from build123d import *

# Parameters (mm, degrees)
BOX021_W     = 19
BOX021_H     = 2
BOX021_DEPTH = 7
BOX020_W     = 19
BOX020_H     = 2
BOX020_DEPTH = 7
BOX018_W     = 1.5
BOX018_H     = 1.5
BOX018_DEPTH = 11.5
BOX016_W     = 1.5
BOX016_H     = 1.5
BOX016_DEPTH = 11.5
BOX017_W     = 1.5
BOX017_H     = 1.5
BOX017_DEPTH = 11.5
BOX019_W     = 1.5
BOX019_H     = 1.5
BOX019_DEPTH = 11.5
BOX015_W     = 5
BOX015_H     = 5
BOX015_DEPTH = 10
BOX013_W     = 1.5
BOX013_H     = 1.5
BOX013_DEPTH = 11.5
BOX011_W     = 1.5
BOX011_H     = 1.5
BOX011_DEPTH = 11.5
BOX012_W     = 1.5
BOX012_H     = 1.5
BOX012_DEPTH = 11.5
BOX014_W     = 1.5
BOX014_H     = 1.5
BOX014_DEPTH = 11.5
BOX010_W     = 5
BOX010_H     = 5
BOX010_DEPTH = 10
BOX023_W     = 19
BOX023_H     = 2
BOX023_DEPTH = 7
BOX003_W     = 1.5
BOX003_H     = 1.5
BOX003_DEPTH = 11.5
BOX001_W     = 1.5
BOX001_H     = 1.5
BOX001_DEPTH = 11.5
BOX002_W     = 1.5
BOX002_H     = 1.5
BOX002_DEPTH = 11.5
BOX004_W     = 1.5
BOX004_H     = 1.5
BOX004_DEPTH = 11.5
BOX_W        = 5
BOX_H        = 5
BOX_DEPTH    = 10
BOX008_W     = 1.5
BOX008_H     = 1.5
BOX008_DEPTH = 11.5
BOX006_W     = 1.5
BOX006_H     = 1.5
BOX006_DEPTH = 11.5
BOX007_W     = 1.5
BOX007_H     = 1.5
BOX007_DEPTH = 11.5
BOX009_W     = 1.5
BOX009_H     = 1.5
BOX009_DEPTH = 11.5
BOX005_W     = 5
BOX005_H     = 5
BOX005_DEPTH = 10
BOX024_W     = 2
BOX024_H     = 3
BOX024_DEPTH = 4
BOX022_W     = 19
BOX022_H     = 2
BOX022_DEPTH = 7


with BuildPart() as cubo021:
    # Box021 → Box021 (new body)
    with BuildSketch(Plane(origin=(0, 5.5, 0), x_dir=(1, 0, 0), z_dir=(0, 0, 1))):
        with Locations((9.5, 1)):
            Rectangle(BOX021_W, BOX021_H)
    extrude(amount=BOX021_DEPTH)


with BuildPart() as cubo020:
    # Box020 → Box020 (new body)
    with BuildSketch(Plane(origin=(18, -10.5, 0), x_dir=(0, 1, 0), z_dir=(0, 0, 1))):
        with Locations((9.5, 1)):
            Rectangle(BOX020_W, BOX020_H)
    extrude(amount=BOX020_DEPTH)


with BuildPart() as cubo018:
    # Box018 → Box018 (new body)
    with BuildSketch(Plane(origin=(3.5, 3.5, 0), x_dir=(1, 0, 0), z_dir=(0, 0, 1))):
        with Locations((0.75, 0.75)):
            Rectangle(BOX018_W, BOX018_H)
    extrude(amount=BOX018_DEPTH)


with BuildPart() as cubo016:
    # Box016 → Box016 (new body)
    with BuildSketch(Plane(origin=(0, 3.5, 0), x_dir=(1, 0, 0), z_dir=(0, 0, 1))):
        with Locations((0.75, 0.75)):
            Rectangle(BOX016_W, BOX016_H)
    extrude(amount=BOX016_DEPTH)


with BuildPart() as cubo017:
    # Box017 → Box017 (new body)
    with BuildSketch(Plane(origin=(3.5, 0, 0), x_dir=(1, 0, 0), z_dir=(0, 0, 1))):
        with Locations((0.75, 0.75)):
            Rectangle(BOX017_W, BOX017_H)
    extrude(amount=BOX017_DEPTH)


with BuildPart() as cubo019:
    # Box019 → Box019 (new body)
    with BuildSketch(Plane.XY):
        with Locations((0.75, 0.75)):
            Rectangle(BOX019_W, BOX019_H)
    extrude(amount=BOX019_DEPTH)


with BuildPart() as fusion015:
    # Box015 → Box015 (new body)
    with BuildSketch(Plane.XY):
        with Locations((2.5, 2.5)):
            Rectangle(BOX015_W, BOX015_H)
    extrude(amount=BOX015_DEPTH)

    # Fusion012: union Cubo019
    add(cubo019.part)

    # Fusion013: union Cubo017
    add(cubo017.part)

    # Fusion014: union Cubo016
    add(cubo016.part)

    # Fusion015: union Cubo018
    add(cubo018.part)


with BuildPart() as fusion015_1:
    # Fusion015 placement: moved
    add(fusion015.part.moved(Location((14, 4, 0))))


with BuildPart() as cubo013:
    # Box013 → Box013 (new body)
    with BuildSketch(Plane(origin=(3.5, 3.5, 0), x_dir=(1, 0, 0), z_dir=(0, 0, 1))):
        with Locations((0.75, 0.75)):
            Rectangle(BOX013_W, BOX013_H)
    extrude(amount=BOX013_DEPTH)


with BuildPart() as cubo011:
    # Box011 → Box011 (new body)
    with BuildSketch(Plane(origin=(0, 3.5, 0), x_dir=(1, 0, 0), z_dir=(0, 0, 1))):
        with Locations((0.75, 0.75)):
            Rectangle(BOX011_W, BOX011_H)
    extrude(amount=BOX011_DEPTH)


with BuildPart() as cubo012:
    # Box012 → Box012 (new body)
    with BuildSketch(Plane(origin=(3.5, 0, 0), x_dir=(1, 0, 0), z_dir=(0, 0, 1))):
        with Locations((0.75, 0.75)):
            Rectangle(BOX012_W, BOX012_H)
    extrude(amount=BOX012_DEPTH)


with BuildPart() as cubo014:
    # Box014 → Box014 (new body)
    with BuildSketch(Plane.XY):
        with Locations((0.75, 0.75)):
            Rectangle(BOX014_W, BOX014_H)
    extrude(amount=BOX014_DEPTH)


with BuildPart() as fusion011:
    # Box010 → Box010 (new body)
    with BuildSketch(Plane.XY):
        with Locations((2.5, 2.5)):
            Rectangle(BOX010_W, BOX010_H)
    extrude(amount=BOX010_DEPTH)

    # Fusion008: union Cubo014
    add(cubo014.part)

    # Fusion009: union Cubo012
    add(cubo012.part)

    # Fusion010: union Cubo011
    add(cubo011.part)

    # Fusion011: union Cubo013
    add(cubo013.part)


with BuildPart() as fusion011_1:
    # Fusion011 placement: moved
    add(fusion011.part.moved(Location((14, -11, 0))))


with BuildPart() as cubo023:
    # Box023 → Box023 (new body)
    with BuildSketch(Plane(origin=(4, -10.5, 0), x_dir=(0, 1, 0), z_dir=(0, 0, 1))):
        with Locations((9.5, 1)):
            Rectangle(BOX023_W, BOX023_H)
    extrude(amount=BOX023_DEPTH)


with BuildPart() as cubo003:
    # Box003 → Box003 (new body)
    with BuildSketch(Plane(origin=(3.5, 3.5, 0), x_dir=(1, 0, 0), z_dir=(0, 0, 1))):
        with Locations((0.75, 0.75)):
            Rectangle(BOX003_W, BOX003_H)
    extrude(amount=BOX003_DEPTH)


with BuildPart() as cubo001:
    # Box001 → Box001 (new body)
    with BuildSketch(Plane(origin=(0, 3.5, 0), x_dir=(1, 0, 0), z_dir=(0, 0, 1))):
        with Locations((0.75, 0.75)):
            Rectangle(BOX001_W, BOX001_H)
    extrude(amount=BOX001_DEPTH)


with BuildPart() as cubo002:
    # Box002 → Box002 (new body)
    with BuildSketch(Plane(origin=(3.5, 0, 0), x_dir=(1, 0, 0), z_dir=(0, 0, 1))):
        with Locations((0.75, 0.75)):
            Rectangle(BOX002_W, BOX002_H)
    extrude(amount=BOX002_DEPTH)


with BuildPart() as cubo004:
    # Box004 → Box004 (new body)
    with BuildSketch(Plane.XY):
        with Locations((0.75, 0.75)):
            Rectangle(BOX004_W, BOX004_H)
    extrude(amount=BOX004_DEPTH)


with BuildPart() as fusion003:
    # Box → Box (new body)
    with BuildSketch(Plane.XY):
        with Locations((2.5, 2.5)):
            Rectangle(BOX_W, BOX_H)
    extrude(amount=BOX_DEPTH)

    # Fusion: union Cubo004
    add(cubo004.part)

    # Fusion001: union Cubo002
    add(cubo002.part)

    # Fusion002: union Cubo001
    add(cubo001.part)

    # Fusion003: union Cubo003
    add(cubo003.part)


with BuildPart() as fusion003_1:
    # Fusion003 placement: moved
    add(fusion003.part.moved(Location((0, 4, 0))))


with BuildPart() as cubo008:
    # Box008 → Box008 (new body)
    with BuildSketch(Plane(origin=(3.5, 3.5, 0), x_dir=(1, 0, 0), z_dir=(0, 0, 1))):
        with Locations((0.75, 0.75)):
            Rectangle(BOX008_W, BOX008_H)
    extrude(amount=BOX008_DEPTH)


with BuildPart() as cubo006:
    # Box006 → Box006 (new body)
    with BuildSketch(Plane(origin=(0, 3.5, 0), x_dir=(1, 0, 0), z_dir=(0, 0, 1))):
        with Locations((0.75, 0.75)):
            Rectangle(BOX006_W, BOX006_H)
    extrude(amount=BOX006_DEPTH)


with BuildPart() as cubo007:
    # Box007 → Box007 (new body)
    with BuildSketch(Plane(origin=(3.5, 0, 0), x_dir=(1, 0, 0), z_dir=(0, 0, 1))):
        with Locations((0.75, 0.75)):
            Rectangle(BOX007_W, BOX007_H)
    extrude(amount=BOX007_DEPTH)


with BuildPart() as cubo009:
    # Box009 → Box009 (new body)
    with BuildSketch(Plane.XY):
        with Locations((0.75, 0.75)):
            Rectangle(BOX009_W, BOX009_H)
    extrude(amount=BOX009_DEPTH)


with BuildPart() as fusion007:
    # Box005 → Box005 (new body)
    with BuildSketch(Plane.XY):
        with Locations((2.5, 2.5)):
            Rectangle(BOX005_W, BOX005_H)
    extrude(amount=BOX005_DEPTH)

    # Fusion004: union Cubo009
    add(cubo009.part)

    # Fusion005: union Cubo007
    add(cubo007.part)

    # Fusion006: union Cubo006
    add(cubo006.part)

    # Fusion007: union Cubo008
    add(cubo008.part)


with BuildPart() as fusion007_1:
    # Fusion007 placement: moved
    add(fusion007.part.moved(Location((0, -11, 0))))


with BuildPart() as cubo024:
    # Box024 → Box024 (new body)
    with BuildSketch(Plane(origin=(8.5, -10, 0), x_dir=(1, 0, 0), z_dir=(0, 0, 1))):
        with Locations((1, 1.5)):
            Rectangle(BOX024_W, BOX024_H)
    extrude(amount=BOX024_DEPTH)


with BuildPart() as fusion016:
    # Box022 → Box022 (new body)
    with BuildSketch(Plane(origin=(0, -9.5, 0), x_dir=(1, 0, 0), z_dir=(0, 0, 1))):
        with Locations((9.5, 1)):
            Rectangle(BOX022_W, BOX022_H)
    extrude(amount=BOX022_DEPTH)

    # Cut: cut Cubo024
    add(cubo024.part, mode=Mode.SUBTRACT)

    # Fusion016: union Cubo021, Cubo020, Fusion015, Fusion011, Cubo023, Fusion003, Fusion007
    add(cubo021.part)
    add(cubo020.part)
    add(fusion015_1.part)
    add(fusion011_1.part)
    add(cubo023.part)
    add(fusion003_1.part)
    add(fusion007_1.part)


solid = fusion016.part
Here's how the part is built. I have some questions about the finished solid (model axes, mm). A direction names the side the tool comes from. Round coordinates to 2 decimals unless told otherwise and drop trailing zeros. Write each loop counter-clockwise with the first axis right and the second up, starting at its lowest first coordinate (ties: lowest second). Pieces come first, ordered by that corner, then holes.
1. Suppose I cut it at A-A (y = 2.5). List the corners of the cut face in (x, z) for me, and give its area (3 significant figures).
2. I need wall thicknesses on L1, parallel to X at y = -5.75, z = 4.25; L2, parallel to Y at x = 15, z = 2.5; L3, parallel to Y at x = 8.25, z = 3. Which ranges of each line are inside material? Lowest first, please.
3. If we mould it in two halves opening along Y, with no side actions, what happens to faces 1 (the flat face through (9, -9, 7)), 2 (the flat face through (15, 7.5, 11)), 3 (the flat face through (2, -11, 6))? For each: released by +Y, released by -Y, zero draft, split by the parting line, or undercut.
4. Will these pins go through, and if not, where does the flat tip stop? pin 1 Ø1.5 at (y, z) = (5.5, 3.5) entering from -X; pin 2 Ø1.5 at (x, y) = (16, 6.5) entering from +Z; pin 3 Ø2 at (x, z) = (8.5, 3.5) entering from -Y; pin 4 Ø5.5 at (y, z) = (-2, 4.5) entering from -X.
5. For faces 4 (the flat face through (3.5, -7, 11)), 5 (the flat face through (15, -7.5, 11)), 6 (the flat face through (19, 6, 6)), which set-ups out of +Z, -Z, +X, -X, +Y, -Y let a thin tool reach every point of the face, with its end or its side?
6. Suppose I cut it at B-B (z = 7.5). List the corners of the cut face in (x, y) for me.
7. Suppose I cut it at C-C (x = 5.75). List the corners of the cut face in (y, z) for me.
Answer sheet:
1. outline: (2, 0) - (4, 0) - (4, 7) - (2, 7) - close; (16, 0) - (18, 0) - (18, 7) - (16, 7) - close
1. area: 28.0 mm2
2. L1: x = 2 to 4, 16 to 18
2. L2: y = -11 to -6, 4 to 9
2. L3: y = -9.5 to -7.5, 5.5 to 7.5
3. face 1: zero draft
3. face 2: undercut
3. face 3: released by -Y
4. pin 1: stops at x = 0
4. pin 2: stops at z = 10
4. pin 3: stops at y = -9.5
4. pin 4: stops at x = 2
5. face 4: +Z, +Y, -Y
5. face 5: +Z, +X, -X
5. face 6: +Z, -Z, +X, +Y, -Y
6. outline: (0, -11) - (5, -11) - (5, -6) - (0, -6) - close; (0, 4) - (5, 4) - (5, 9) - (0, 9) - close; (14, -11) - (19, -11) - (19, -6) - (14, -6) - close; (14, 4) - (19, 4) - (19, 9) - (14, 9) - close
7. outline: (-9.5, 0) - (-7.5, 0) - (-7.5, 7) - (-9.5, 7) - close; (5.5, 0) - (7.5, 0) - (7.5, 7) - (5.5, 7) - close
